Verification items for the finished model (mm, model axes). Face numbers are marked on the shaded views. A direction names the side the tool comes from. Coordinates: 2 decimals unless noted, no trailing zeros. Order: outer loops, then holes, each group sorted by start corner. A loop starts at its lowest first (then second) coordinate and runs counter-clockwise, first axis right, second up. Notation, with made-up numbers: M 34.25,15.25 L 58.25,15.25 A28 cw 58.25,38.25 Z; hole C 75,84.25 d6. An arc over 180 degrees is marked long. Return JSON: item names as keys, results as strings. Group by question number.
1. Section check B-B, the plane z = 10.75. Record the cut outline in (x, y).
2. Section check C-C, the plane x = 58. Record the cut outline in (y, z).
3. Gauge pin test, flat end, axial feed: pin 1 (18 mm diameter, centred on x = 31.5, y = 19, fed in from +Z). Record the tip position at first contact, or that the pin passes through.
4. Material ranges on line 1 along X through (y, z) = (8, 5.25); line 2 along Y through (x, z) = (47, 9.75); line 3 along Z through (x, y) = (73, 29), recorded low to high.
5. Mould release check, pull along X, two halves, no side actions. Record for the marked faces 3, 4 and 5: +X half, -X half, draft (parallel to the pull), parting line (faces both ways), or undercut.
6. Section check A-A, the plane y = 26.5. Record the cut outline in (x, z).
7. Set-up check for the marked faces 1 and 2: record each of +Z, -Z, +X, -X, +Y, -Y from which the full face is reachable in a straight line by a thin tool's end or side.
```python
from build123d import *

# Parameters (mm, degrees)
F0_W     = 96.52
F0_H     = 62.23
F1_DEPTH = 15.24
F2_R     = 3.81
F3_R     = 3.81
F4_R     = 3.81
F5_R     = 3.81
F6_W     = 93.98
F6_H     = 59.69
F7_DEPTH = 12.954
F8_R     = 3.81
F9_R     = 3.81


with BuildPart() as f1:
    # F0 (on Top) → F1 (new body)
    with BuildSketch(Plane.XY):
        with Locations((29.339396, 19.943792)):
            Rectangle(F0_W, F0_H)
    extrude(amount=F1_DEPTH)

    # F2
    f2_edges = [f1.edges().sort_by_distance(p)[0] for p in [
        (-18.920604, -11.171208, 7.62),
    ]]
    fillet(f2_edges, radius=F2_R)

    # F3
    f3_edges = [f1.edges().sort_by_distance(p)[0] for p in [
        (77.599396, -11.171208, 7.62),
    ]]
    fillet(f3_edges, radius=F3_R)

    # F4
    f4_edges = [f1.edges().sort_by_distance(p)[0] for p in [
        (77.599396, 51.058792, 7.62),
    ]]
    fillet(f4_edges, radius=F4_R)

    # F5
    f5_edges = [f1.edges().sort_by_distance(p)[0] for p in [
        (-18.920604, 51.058792, 7.62),
    ]]
    fillet(f5_edges, radius=F5_R)

    # F6 (on face) → F7 (cut)
    with BuildSketch(Plane.XY.offset(15.24)):
        with Locations((29.339396, 19.943792)):
            Rectangle(F6_W, F6_H)
    extrude(amount=-F7_DEPTH, mode=Mode.SUBTRACT)

    # F8
    f8_edges = [f1.edges().sort_by_distance(p)[0] for p in [
        (-17.650604, 49.788792, 8.763),
    ]]
    fillet(f8_edges, radius=F8_R)

    # F9
    f9_edges = [f1.edges().sort_by_distance(p)[0] for p in [
        (76.329396, 49.788792, 8.763),
        (-17.650604, -9.901208, 8.763),
        (76.329396, -9.901208, 8.763),
    ]]
    fillet(f9_edges, radius=F9_R)


solid = f1.part
```
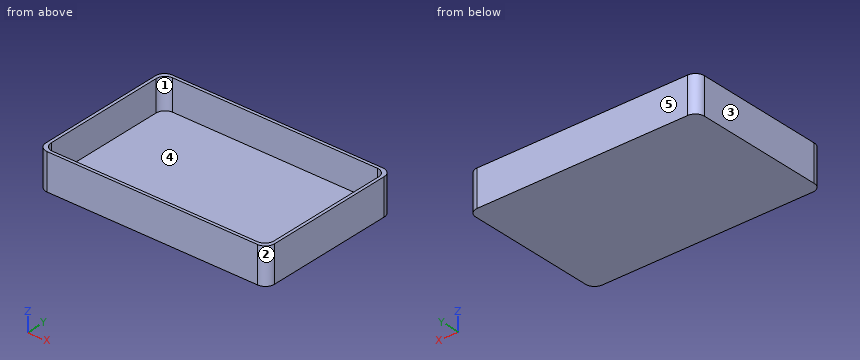
Answers follow:
{
 "1": {"outline": "M -18.92,-7.36 A3.81 ccw -15.11,-11.17 L 73.79,-11.17 A3.81 ccw 77.6,-7.36 L 77.6,47.25 A3.81 ccw 73.79,51.06 L -15.11,51.06 A3.81 ccw -18.92,47.25 Z; hole M -17.65,-6.09 A3.81 ccw -13.84,-9.9 L 72.52,-9.9 A3.81 ccw 76.33,-6.09 L 76.33,45.98 A3.81 ccw 72.52,49.79 L -13.84,49.79 A3.81 ccw -17.65,45.98 Z"},
 "2": {"outline": "M -11.17,0 L 51.06,0 L 51.06,15.24 L 49.79,15.24 L 49.79,2.29 L -9.9,2.29 L -9.9,15.24 L -11.17,15.24 Z"},
 "3": {"pin 1": "z = 2.29"},
 "4": {"line 1": "-18.92 to -17.65, 76.33 to 77.6", "line 2": "-11.17 to -9.9, 49.79 to 51.06", "line 3": "0 to 2.29"},
 "5": {"face 3": "-X half", "face 4": "undercut", "face 5": "draft"},
 "6": {"outline": "M -18.92,0 L 77.6,0 L 77.6,15.24 L 76.33,15.24 L 76.33,2.29 L -17.65,2.29 L -17.65,15.24 L -18.92,15.24 Z"},
 "7": {"face 1": "+Z", "face 2": "+Z, -Z, +X, -Y"}
}
